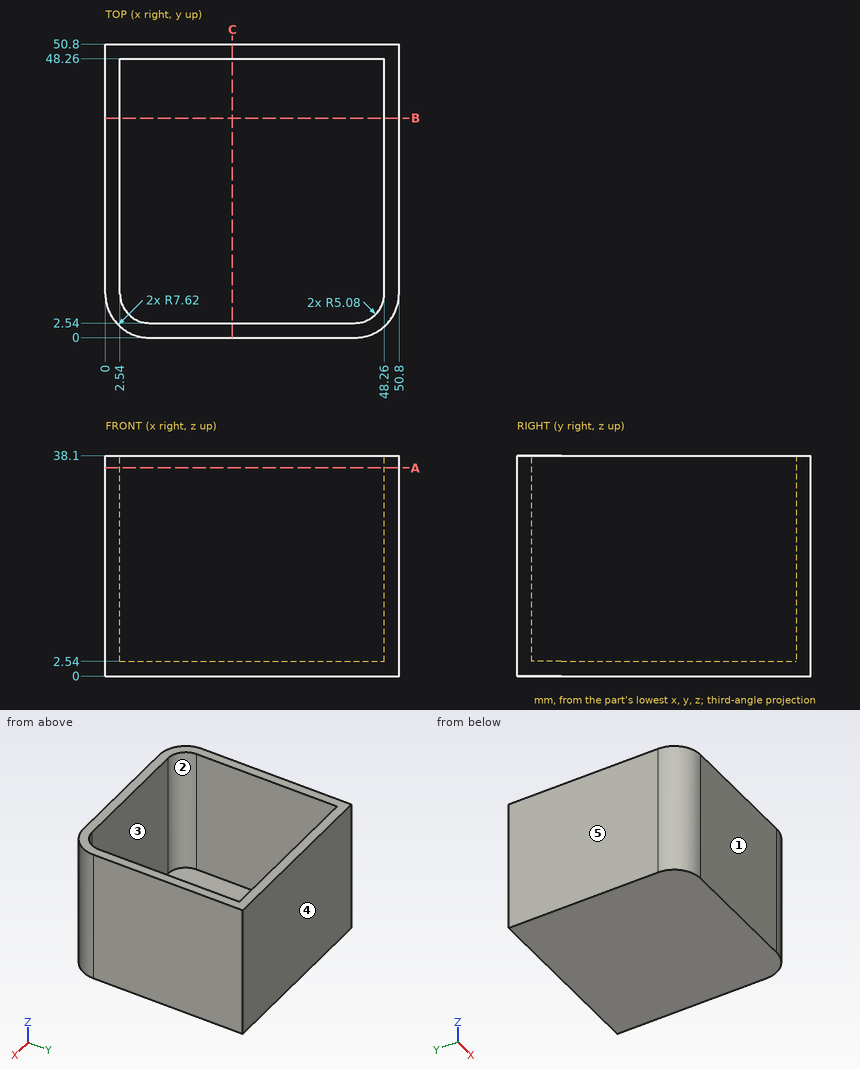
The figure shows three views and two pictorial views of one solid part (mm, origin at its lowest corner). Answer the questions. A direction names the side the tool comes from. Round coordinates to 2 decimals unless told otherwise and drop trailing zeros. Write each loop counter-clockwise with the first axis right and the second up, starting at its lowest first coordinate (ties: lowest second). Pieces come first, ordered by that corner, then holes. Notation, with made-up numbers: (27, 53.5) - (38, 53.5) arc R16 ccw to (38, 82.5) - close; hole circle Ø8 at (85.5, 40.5). An arc over 180 degrees is marked (long way). One line per question, with ' | ' between items. Start each with the question number.
1. Section A-A (z = 36) is taken. Determine the outline of the cut face in (x, y).
2. Find the intervals of material crossed by probe 1 along X at (y, z) = (38.5, 20); probe 2 along Z at (x, y) = (36.5, 38.5), in increasing order. Write a range as [from, to].
3. Section B-B (y = 38) is taken. Determine the outline of the cut face in (x, z).
4. For the marked faces 1 and 2, determine the directions among +Z, -Z, +X, -X, +Y, -Y from which every point of the face is accessible in a straight line to the end or side of a thin tool.
5. Each of these flat-tipped pins is pushed along its axis until it touches: pin 1 (12 mm diameter, centred on x = 37.5, y = 23, fed in from +Z); pin 2 (1.5 mm diameter, centred on y = 6.5, z = 28.5, fed in from +X). Where does it stop, or does it pass through?
6. For a pull along X with two mould halves and no side action, classify the marked faces 3, 4 and 5 as +X half, -X half, draft (parallel to the pull), parting line (faces both ways), or undercut.
Filled in:
1) outline: (0, 7.62) arc R7.62 ccw to (7.62, 0) - (43.18, 0) arc R7.62 ccw to (50.8, 7.62) - (50.8, 50.8) - (0, 50.8) - close; hole (2.54, 7.62) arc R5.08 ccw to (7.62, 2.54) - (43.18, 2.54) arc R5.08 ccw to (48.26, 7.62) - (48.26, 48.26) - (2.54, 48.26) - close
2) probe 1: [0, 2.54], [48.26, 50.8] | probe 2: [0, 2.54]
3) outline: (0, 0) - (50.8, 0) - (50.8, 38.1) - (48.26, 38.1) - (48.26, 2.54) - (2.54, 2.54) - (2.54, 38.1) - (0, 38.1) - close
4) face 1: +Z, -Z, +X, -X, -Y | face 2: +Z
5) pin 1: z = 2.54 | pin 2: x = 50.79
6) face 3: undercut | face 4: draft | face 5: -X half
